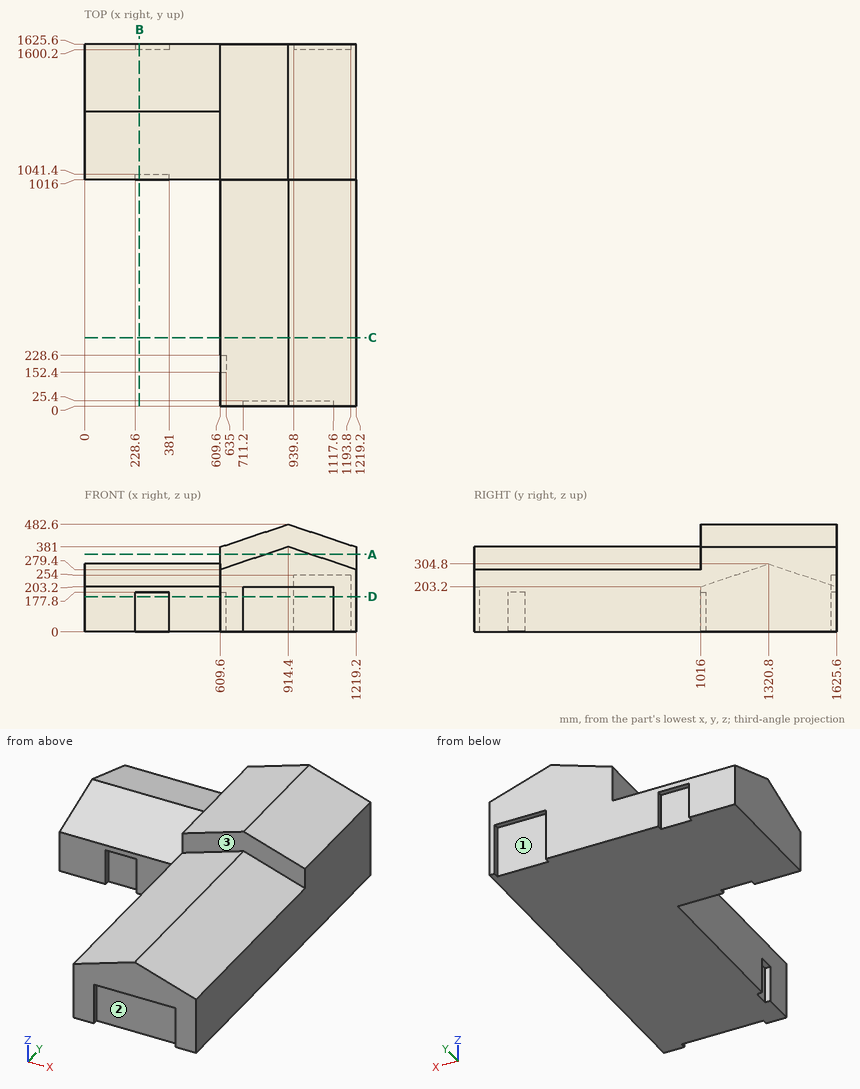
Study the drawing (mm; zero at the part's minimum x, y, z) and answer. A direction names the side the tool comes from. Round coordinates to 2 decimals unless told otherwise and drop trailing zeros. Write each loop counter-clockwise with the first axis right and the second up, starting at its lowest first coordinate (ties: lowest second). Pieces come first, ordered by that corner, then holes. Notation, with made-up numbers: (70, 13) - (96, 13) arc R12 cw to (96, 17) - close; hole circle Ø5 at (86, 76). An arc over 180 degrees is marked (long way). Use a Markdown table: item, result. Add a question column.
1. The part is cut by section A-A (z = 348). Write down the section's boundary in (x, y).
2. A tool of negligible diameter and unlimited length cuts with its end or side. For the marked faces 1, 2 and 3, from which of +Z, -Z, +X, -X, +Y, -Y can it reach the whole face along a straight path? Write none if from no direction.
3. The part is cut by section C-C (y = 308). Write down the section's boundary in (x, z).
4. The part is cut by section D-D (z = 158). Write down the section's boundary in (x, y), and give its area (3 significant figures).
5. The part is cut by section B-B (x = 246). Write down the section's boundary in (y, z), and give its area (3 significant figures).
6. Consider line 1 (X direction, y = 344.5, z = 201); line 2 (Y direction, x = 882.5, z = 440); line 3 (Y direction, x = 1136, z = 159.5). Determine where each line is inside the solid, lowest interval first.
7. Flat-ended cylindrical pins translate along their axes: P1, Ø12.5, axis at x = 306, y = 1614, coming from the -Z side; P2, Ø1.5, axis at y = 886, z = 71.5, coming from the -X side; P3, Ø6, axis at x = 489.5, y = 1166.5, coming from the +Z side; P4, Ø7.5, axis at x = 628.5, z = 111, coming from the -Y side. Find the tip coordinate at first contact, or state that the pin passes through.
Reported:
| question | item | result |
|---|---|---|
| 1 | outline | (609.6, 1016) - (815.4, 1016) - (815.4, 0) - (1013.4, 0) - (1013.4, 1016) - (1219.2, 1016) - (1219.2, 1625.6) - (609.6, 1625.6) - close |
| 2 | face 1 | -Z, +Y |
| 2 | face 2 | -Z, -Y |
| 2 | face 3 | +Z, -Y |
| 3 | outline | (609.6, 0) - (1219.2, 0) - (1219.2, 279.4) - (914.4, 381) - (609.6, 279.4) - close |
| 4 | outline | (0, 1016) - (228.6, 1016) - (228.6, 1041.4) - (381, 1041.4) - (381, 1016) - (609.6, 1016) - (609.6, 228.6) - (635, 228.6) - (635, 152.4) - (609.6, 152.4) - (609.6, 0) - (711.2, 0) - (711.2, 25.4) - (1117.6, 25.4) - (1117.6, 0) - (1219.2, 0) - (1219.2, 1625.6) - (1193.8, 1625.6) - (1193.8, 1600.2) - (939.8, 1600.2) - (939.8, 1625.6) - (381, 1625.6) - (381, 1600.2) - (228.6, 1600.2) - (228.6, 1625.6) - (0, 1625.6) - close |
| 4 | area | 1,340,000 mm^2 |
| 5 | outline | (1016, 177.8) - (1041.4, 177.8) - (1041.4, 0) - (1600.2, 0) - (1600.2, 177.8) - (1625.6, 177.8) - (1625.6, 203.2) - (1320.8, 304.8) - (1016, 203.2) - close |
| 5 | area | 146,000 mm^2 |
| 6 | line 1 | 609.6 to 1219.2 |
| 6 | line 2 | 1016 to 1625.6 |
| 6 | line 3 | 0 to 1600.2 |
| 7 | P1 | z = 177.8 |
| 7 | P2 | x = 609.6 |
| 7 | P3 | z = 254.37 |
| 7 | P4 | y = 0 |
